The listing builds one solid part. Answer for the finished solid, in the listing's coordinates (mm). A direction names the side the tool comes from. Round coordinates to 2 decimals unless told otherwise and drop trailing zeros. Write each loop counter-clockwise with the first axis right and the second up, starting at its lowest first coordinate (ties: lowest second). Pieces come first, ordered by that corner, then holes.
(1) The mould has two halves that part along X. Classify faces 3 (the face through (47.16, -1.08, -4.88)), 4 (the face through (93.2, 0, 0)), 5 (the face through (6.06, 2.58, 4.05)): +X half, -X half, draft (parallel to the pull), parting line (faces both ways), or undercut.
(2) A cutting plane is placed at A-A, the plane x = 36.5. Give the vertices of the cut face in (y, z).
(3) For faces 1 (the face through (90.24, -1.08, -4.88)), 2 (the face through (87.16, 2.58, 4.05)), determine the directions among +Z, -Z, +X, -X, +Y, -Y from which every point of the face is accessible in a straight line to the end or side of a thin tool.
(4) Each of these flat-tipped pins is pushed along its axis until it touches: pin 1 Ø2 at (x, z) = (57.5, -1.5) entering from +Y; pin 2 Ø2 at (x, z) = (64.5, -2.5) entering from -Y; pin 3 Ø2 at (x, z) = (21, 2) entering from +Y. Where does it stop, or does it pass through?
(5) Find the intervals of material crossed by probe 1 along Z at (x, y) = (27, 0.25); probe 2 along Z at (x, y) = (50.5, -1.25), in increasing order.
Autodesk Inventor part; units mm, degrees
ref_plane "YZ Plane" through (0, 0, 0) normal (1, 0, 0) x (0, 1, 0)
ref_plane "XZ Plane" through (0, 0, 0) normal (0, 1, 0) x (-1, 0, 0)
sketch "Skizze1" plane through (0, 0, 0) normal (0, 0, 1) x (1, 0, 0)
  line L0 (0, 0) -> (0, 5)
  line L1 (93.2, 5) -> (93.2, 0)
  line L2 (93.2, 0) -> (0, 0)
  line L3 (5.5, 5) -> (5.5, 4.8)
  line L4 (5.5, 4.8) -> (6.6, 4.8)
  line L5 (6.6, 4.8) -> (6.6, 5)
  line L6 (0, 5) -> (5.5, 5)
  line L7 (86.6, 5) -> (86.6, 4.8)
  line L8 (86.6, 4.8) -> (87.7, 4.8)
  line L9 (87.7, 4.8) -> (87.7, 5)
  line L10 (6.6, 5) -> (86.6, 5)
  line L11 (87.7, 5) -> (93.2, 5)
  line L12 (46.6, 0) -> (46.6, 5) construction
  line L13 (0.5, 5) -> (0.5, 0) construction
  line L14 (92.7, 5) -> (92.7, 0) construction
  line L15 (15.6, 0) -> (15.6, 5) construction
  line L16 (77.6, 0) -> (77.6, 5) construction
  line L17 (28.6, 5) -> (28.6, 0) construction
  line L18 (64.6, 5) -> (64.6, 0) construction
  dimension "d2" = 10
  dimension "d3" = 9.6
  dimension "d4" = 1.1
  dimension "d6" = 1.1
  dimension "d8" = 82.2
  dimension "d9" = 5
  dimension "d10" = 5
  dimension "d11" = 0.5
  dimension "d12" = 93.2
  dimension "d16" = 31
  dimension "d17" = 62
  dimension "d18" = 13
  dimension "d19" = 13
revolve "Umdrehung1" add sketch "Skizze1" angle 360 about axis through (93.2, 0, 0) along (-1, 0, 0)
sketch "Skizze2" plane through (46.6, 0, 5) normal (0, 0, 1) x (1, 0, 0)
  line L0 (-31, 0) -> (-31, 5) construction
  line L1 (-18, 5) -> (-18, 0) construction
  line L2 (18, 5) -> (18, 0) construction
  line L3 (31, 0) -> (31, 5) construction
  line L4 (-31, 5) -> (-18, 5)
  line L5 (-18, 5) -> (-18, -5)
  line L6 (-18, -5) -> (-31, -5)
  line L7 (-31, -5) -> (-31, 5)
  line L8 (18, 5) -> (31, 5)
  line L9 (31, 5) -> (31, -5)
  line L10 (31, -5) -> (18, -5)
  line L11 (18, -5) -> (18, 5)
  point P0 (-46.6, 0)
  dimension "d20" = 10
  dimension "d21" = 10
chamfer "Fase1" distance 0.5 angle 45 2 edges at (0, -5, 0) (93.2, -5, 0)
ref_plane "Arbeitsebene1" through (46.6, 0, 5) normal (0, 0, 1) x (1, 0, 0)
equation "\"d20\" = d2"
equation "\"d21\" = d20"
equation "\"d6\" = d4"
equation "\"d10\" = d9"
equation "\"d19\" = d18"
properties part number "ParallelMecha_DrivenShaft" material "Edelstahl"
Solutions:
1. face 3: draft
1. face 4: +X half
1. face 5: undercut
2. outline: circle Ø10 at (0, 0)
3. face 1: +X, -X
3. face 2: none
4. pin 1: stops at y = 4.97
4. pin 2: stops at y = -4.77
4. pin 3: stops at y = 4.9
5. probe 1: z = -4.99 to 4.99
5. probe 2: z = -4.84 to 4.84
